```python
from build123d import *

# Parameters (mm, degrees)
SKETCH_1_R      = 3
EXTRUDE_1_DEPTH = 16
CHAMFER_1_SIZE  = 0.5


with BuildPart() as part:
    # 草图1 → 凸台-拉伸1 (new body)
    with BuildSketch(Plane(origin=(0, 0, 0), x_dir=(1, 0, 0), z_dir=(0, 1, 0))):
        with BuildLine():
            ThreePointArc((-5.240891545, 36.838305804), (1.458305804, 40.620891545), (5.240891545, 33.921694196))
            ThreePointArc((5.240891545, 33.921694196), (3.024711954, 17.69), (5.240891545, 1.458305804))
            ThreePointArc((5.240891545, 1.458305804), (1.458305804, -5.240891545), (-5.240891545, -1.458305804))
            ThreePointArc((-5.240891545, -1.458305804), (-7.855288046, 17.69), (-5.240891545, 36.838305804))
        make_face()
        Circle(SKETCH_1_R, mode=Mode.SUBTRACT)
        with Locations((0, 35.38)):
            Circle(SKETCH_1_R, mode=Mode.SUBTRACT)
    extrude(amount=EXTRUDE_1_DEPTH)

    # 倒角1
    chamfer_1_edges = [part.edges().sort_by_distance(p)[0] for p in [
        (3.024711954, 16, -17.69),
        (1.458305804, 16, -40.620891545),
        (-7.855288046, 16, -17.69),
        (1.458305804, 0, -40.620891545),
        (3.024711954, 0, -17.69),
        (1.458305804, 0, 5.240891545),
        (-7.855288046, 0, -17.69),
        (1.458305804, 16, 5.240891545),
    ]]
    chamfer(chamfer_1_edges, length=CHAMFER_1_SIZE)


solid = part.part
```
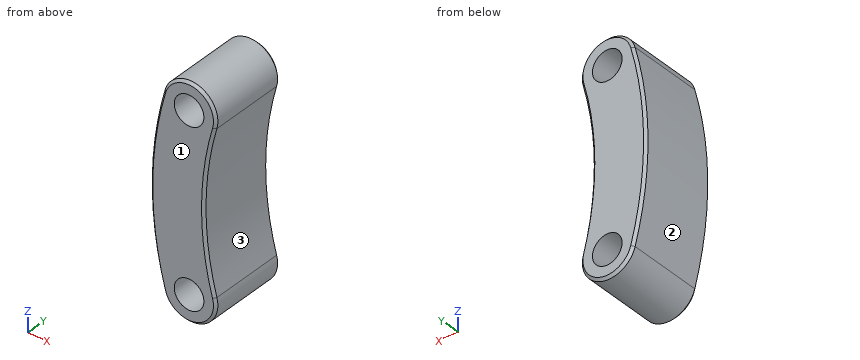
Model file for the job. Use its own axes, mm. Face numbers are marked on the shaded views. Coordinates: 2 decimals unless noted, no trailing zeros. Order: outer loops, then holes, each group sorted by start corner. A loop starts at its lowest first (then second) coordinate and runs counter-clockwise, first axis right, second up. Notation, with made-up numbers: (88, 9.5) -> (103, 9.5) arc R19 cw to (103, 17.5) -> close; hole circle Ø7 at (20, 51). An arc over 180 degrees is marked (long way). Answer as a JSON object with one key per item and string values. Group by question number.
1) Cut at A-A, the plane x = 0. Write the cut outline in (y, z).
2) Cut at B-B, the plane y = 12.5. Write the cut outline in (x, z).
3) Drill centre lines: L1, parallel to Z at x = 0, y = 9; L2, parallel to Z at x = 2.25, y = 9; L3, parallel to Y at x = -3.5, z = 3.5. Where is each one in solid material? Low to high.
4) Pull direction Z, two halves, no side cores. Call the marked faces 1, 2 and 3: +Z half, -Z half, draft (parallel to the pull), parting line (faces both ways), or undercut.
5) Flat gauge pins, fed straight in: pin 1 (2 mm diameter, centred on x = -4.5, y = 14, fed in from -Z); pin 2 (5 mm diameter, centred on x = -2, y = 12, fed in from +Z); pin 3 (5 mm diameter, centred on y = 8.5, z = -32.5, fed in from -X). Where does each tip first touch, or does it go through?
Check values:
{
 "1": {"outline": "(0, -40.32) -> (0.5, -40.82) -> (15.5, -40.82) -> (16, -40.32) -> (16, -38.38) -> (0, -38.38) -> close; (0, -32.38) -> (16, -32.38) -> (16, -3) -> (0, -3) -> close; (0, 3) -> (16, 3) -> (16, 4.94) -> (15.5, 5.44) -> (0.5, 5.44) -> (0, 4.94) -> close"},
 "2": {"outline": "(-5.24, -36.84) arc R5.44 ccw to (5.24, -33.92) arc R60.55 cw to (5.24, -1.46) arc R5.44 ccw to (-5.24, 1.46) arc R71.43 ccw to start; hole circle Ø6 at (0, -35.38); hole circle Ø6 at (0, 0)"},
 "3": {"L1": "z = -40.82 to -38.38, -32.38 to -3, 3 to 5.44", "L2": "z = -40.33 to -37.36, -33.4 to -1.98, 1.98 to 4.95", "L3": "y = 0.01 to 15.99"},
 "4": {"face 1": "draft", "face 2": "parting line", "face 3": "undercut"},
 "5": {"pin 1": "stops at z = -39.54", "pin 2": "stops at z = 5.44", "pin 3": "stops at x = -6.79"}
}
